Read the model definition and answer for the solid it produces. Units are mm, in the model's axes. A direction names the side the tool comes from. Round coordinates to 2 decimals unless told otherwise and drop trailing zeros. Order: outer loops, then holes, each group sorted by start corner. A loop starts at its lowest first (then second) coordinate and runs counter-clockwise, first axis right, second up. Notation, with made-up numbers: (64.25, 3) - (77.25, 3) arc R15 cw to (77.25, 26) - close; hole circle Ø10 at (9, 53.25). An arc over 180 degrees is marked (long way). Put each result on its own line as item: value. Start each with the question number.
Q1. For a pull along Z with two mould halves and no side action, classify faces 5 (the face through (0, 1.651, 13)), 6 (the face through (12.088, 4.057, 1.587)), 7 (the face through (-5.142, 0.837, 9.879)), 8 (the face through (-0.09, 0.84, 13.97)) as pulls with the +Z half, pulls with the -Z half, needs draft (parallel to the pull), parting line crosses it, or undercut.
Q2. Which of the six approach directions +Z, -Z, +X, -X, +Y, -Y give full straight-line access (tool end or side, diameter ignored) to faces 1 (the face through (12.5, 2.54, -2.1)), 2 (the face through (0, 3.556, 0)), 3 (the face through (5.18, 0.84, 9.95)), 4 (the face through (-6.497, 0.837, 1.443))?
Q3. Section C-C on x = 0 is taken. Give the vertices of the cut face in (y, z) (3 decimals), then the cut area to 3 significant figures.
Q4. Section D-D on y = 3.15 is taken. Give the vertices of the cut face in (x, z).
Q5. Each of these flat-tipped pins is pushed along its axis until it touches: pin 1 Ø1.5 at (y, z) = (1.5, 7.5) entering from -X; pin 2 Ø6 at (x, z) = (7.5, -7.5) entering from -Y. Where does it stop, or does it pass through?
Q6. Section A-A on y = 0.8 is taken. Give the vertices of the cut face in (x, z), then the cut area to 3 significant figures.
Q7. Section B-B on z = 0 is taken. Give the vertices of the cut face in (x, y) (3 decimals).
Q8. Find the intervals of material crossed by line 1 along X through (y, z) = (4.15, 0); line 2 along Y through (x, z) = (5.75, 10.5); line 3 along Y through (x, z) = (2.5, 13), in increasing order. Write a range as from..to.
from build123d import *

# Parameters (mm, degrees)
BOSS_EXTRUDE1_DEPTH = 1.651


with BuildPart() as part:
    # Sketch1 → Revolve1 (revolve)
    with BuildSketch(Plane(origin=(0, 0, 0), x_dir=(0, 0, -1), z_dir=(1, 0, 0))):
        Polygon((0, 0), (6.6548, 0), (6.6548, 1.651), (12.5222, 1.651), (12.5222, 2.54), (13.97, 2.54), (13.97, 4.318), (13.335, 4.318), (13.335, 4.572), (12.192, 4.572), (12.192, 3.556), (0, 3.556), align=None)
    revolve(axis=Axis((0, 3.556, 0), (0, -1, 0)))

    # Sketch2 → Boss-Extrude1 (add)
    with BuildSketch(Plane.XZ.offset(-1.651)):
        with BuildLine():
            Line((-3.870376876, 7.434924804), (-6.450628127, 12.391541339))
            ThreePointArc((-6.450628127, 12.391541339), (0, 13.97), (6.450628127, 12.391541339))
            Line((6.450628127, 12.391541339), (3.870376876, 7.434924804))
            ThreePointArc((3.870376876, 7.434924804), (0, 8.382), (-3.870376876, 7.434924804))
        make_face()
    extrude(amount=BOSS_EXTRUDE1_DEPTH)


solid = part.part
Findings:
1. face 5: needs draft
1. face 6: undercut
1. face 7: undercut
1. face 8: pulls with the +Z half
2. face 1: none
2. face 2: +Y
2. face 3: +X, -Y
2. face 4: -Y
3. outline: (0, -6.655) - (1.651, -6.655) - (1.651, -12.522) - (2.54, -12.522) - (2.54, -13.97) - (4.318, -13.97) - (4.318, -13.335) - (4.572, -13.335) - (4.572, -12.192) - (3.556, -12.192) - (3.556, 12.192) - (4.572, 12.192) - (4.572, 13.335) - (4.318, 13.335) - (4.318, 13.97) - (2.54, 13.97) - (2.54, 12.522) - (1.651, 12.522) - (1.651, 13.97) - (0, 13.97) - (0, 8.382) - (1.651, 8.382) - (1.651, 6.655) - (0, 6.655) - close
3. area: 85.1 mm2
4. outline: circle Ø27.94 at (0, 0)
5. pin 1: x = -10.54
5. pin 2: y = 1.65
6. outline: circle Ø13.31 at (0, 0); (-6.45, 12.39) - (-3.87, 7.43) arc R8.38 cw to (3.87, 7.43) - (6.45, 12.39) arc R13.97 ccw to start
6. area: 199 mm2
7. outline: (-13.97, 2.54) - (-12.522, 2.54) - (-12.522, 1.651) - (-6.655, 1.651) - (-6.655, 0) - (6.655, 0) - (6.655, 1.651) - (12.522, 1.651) - (12.522, 2.54) - (13.97, 2.54) - (13.97, 4.318) - (13.335, 4.318) - (13.335, 4.572) - (12.192, 4.572) - (12.192, 3.556) - (-12.192, 3.556) - (-12.192, 4.572) - (-13.335, 4.572) - (-13.335, 4.318) - (-13.97, 4.318) - close
8. line 1: -13.97..-12.19, 12.19..13.97
8. line 2: 1.65..3.56
8. line 3: 0..1.65, 2.54..4.57
